from build123d import *

# Parameters (mm, degrees)
EXTRUDE_1_DEPTH = 100


with BuildPart() as part:
    # 草图1 → 凸台-拉伸1 (new, symmetric)
    with BuildSketch(Plane(origin=(0, 0, 0), x_dir=(0, 0, -1), z_dir=(1, 0, 0))):
        with BuildLine():
            Line((-1.5, 14.924811557), (-1.5, 0))
            Line((-1.5, 0), (1.5, 0))
            Line((1.5, 0), (1.5, 14.924811557))
            ThreePointArc((1.5, 14.924811557), (0, 15), (-1.5, 14.924811557))
        make_face()
        with BuildLine():
            Line((1.5, 0), (-1.5, 0))
            Line((-1.5, 0), (-1.5, 14.924811557))
            ThreePointArc((-1.5, 14.924811557), (-10.062305899, -11.124297731), (15, 0))
            ThreePointArc((15, 0), (11.124297731, 10.062305899), (1.5, 14.924811557))
            Line((1.5, 14.924811557), (1.5, 0))
        make_face()
        with BuildLine():
            Line((-1.5, 17), (-1.5, 14.924811557))
            ThreePointArc((-1.5, 14.924811557), (0, 15), (1.5, 14.924811557))
            Line((1.5, 14.924811557), (1.5, 17))
            Line((1.5, 17), (-1.5, 17))
        make_face()
    extrude(amount=EXTRUDE_1_DEPTH, both=True)


solid = part.part
CAD build for the part. Positions are in the model's coordinates, mm. Coordinates: 2 decimals unless noted, no trailing zeros. Write each loop counter-clockwise with the first axis right and the second up, starting at its lowest first coordinate (ties: lowest second). Pieces come first, ordered by that corner, then holes. Notation, with made-up numbers: (51, 71.5) - (69, 71.5) arc R28 cw to (69, 100.5) - close; hole circle Ø2 at (35, 87). An arc over 180 degrees is marked (long way). Use a Markdown table: item, result. Add a question column.
Item 1: Band-saw the part on B-B, the plane y = 12. Give the cut face in (x, z).
Item 2: Drill centre lines: L1, parallel to Z at x = -25, y = 15.5; L2, parallel to Y at x = -0.5, z = -1; L3, parallel to Z at x = -0.5, y = 2. Where is each one in solid material? Low to high. Write a range as from..to.
Item 3: Band-saw the part on A-A, the plane x = 69. Give the cut face in (y, z), and give its area (3 significant figures).
Item 4: Flat gauge pins, fed straight in: pin 1 (3 mm diameter, centred on x = 52, z = 9.5, fed in from +Y); pin 2 (2 mm diameter, centred on x = -47, z = -11.5, fed in from -Y); pin 3 (1 mm diameter, centred on x = -13, y = 10, fed in from +Z). Where does each tip first touch, or does it go through?
Item 5: Band-saw the part on C-C, the plane z = 6.5. Give the cut face in (x, y), and give its area (3 significant figures).
Numbers:
| question | item | result |
|---|---|---|
| 1 | outline | (-100, -9) - (100, -9) - (100, 9) - (-100, 9) - close |
| 2 | L1 | -1.5..1.5 |
| 2 | L2 | -14.97..17 |
| 2 | L3 | -14.87..14.87 |
| 3 | outline | (14.92, -1.5) - (17, -1.5) - (17, 1.5) - (14.92, 1.5) arc R15 ccw (long way) to start |
| 3 | area | 713 mm2 |
| 4 | pin 1 | y = 12.69 |
| 4 | pin 2 | y = -10.71 |
| 4 | pin 3 | z = 11.61 |
| 5 | outline | (-100, -13.52) - (100, -13.52) - (100, 13.52) - (-100, 13.52) - close |
| 5 | area | 5,410 mm2 |
